from build123d import *

# Parameters (mm, degrees)
EXTRUDE1_DEPTH             = 500
SKETCH2_R                  = 1.75
EXTRUDE2_DEPTH             = 6.5
SKETCH_R                   = 3
SKETCH_R_2                 = 1.75
EXTRUDE4_DEPTH             = 3.5
CHAMFER1_SIZE              = 0.2
LPATTERN1_COUNT            = 24
LPATTERN1_PITCH            = 20
CHAMFER1_OF_LPATTERN1_SIZE = 0.2


with BuildPart() as part:
    # Sketch1 → Extrude1 (new body)
    with BuildSketch(Plane.XY):
        with BuildLine():
            Line((-4.3, -3.25), (4.3, -3.25))
            Line((4.3, -3.25), (4.5, -3.05))
            Line((4.5, -3.05), (4.5, 0.455012563))
            ThreePointArc((4.5, 0.455012563), (3.924845827, 0.712323349), (3.617735397, 1.2625))
            Line((3.617735397, 1.2625), (3.15008224, 1.2625))
            Line((3.15008224, 1.2625), (3.15008224, 1.7625))
            Line((3.15008224, 1.7625), (3.65008224, 1.7625))
            ThreePointArc((3.65008224, 1.7625), (3.973877727, 2.229724887), (4.5, 2.444987437))
            Line((4.5, 2.444987437), (4.5, 3.05))
            Line((4.5, 3.05), (4.3, 3.25))
            Line((4.3, 3.25), (-4.3, 3.25))
            Line((-4.3, 3.25), (-4.5, 3.05))
            Line((-4.5, 3.05), (-4.5, 2.444987437))
            ThreePointArc((-4.5, 2.444987437), (-3.973877727, 2.229724887), (-3.65008224, 1.7625))
            Line((-3.65008224, 1.7625), (-3.15008224, 1.7625))
            Line((-3.15008224, 1.7625), (-3.15008224, 1.2625))
            Line((-3.15008224, 1.2625), (-3.617735397, 1.2625))
            ThreePointArc((-3.617735397, 1.2625), (-3.924845827, 0.712323349), (-4.5, 0.455012563))
            Line((-4.5, 0.455012563), (-4.5, -3.05))
            Line((-4.5, -3.05), (-4.3, -3.25))
        make_face()
    extrude(amount=EXTRUDE1_DEPTH)

    # Sketch2 → Extrude2 (cut)
    with BuildSketch(Plane(origin=(0, 3.25, 0), x_dir=(1, 0, 0), z_dir=(0, 1, 0))):
        with Locations((0, -15)):
            Circle(SKETCH2_R)
    extrude2 = extrude(amount=-EXTRUDE2_DEPTH, mode=Mode.SUBTRACT)

    # Sketch → Extrude4 (cut)
    with BuildSketch(Plane(origin=(0, 3.25, 0), x_dir=(1, 0, 0), z_dir=(0, 1, 0))):
        with Locations((0, -15)):
            Circle(SKETCH_R)
        with Locations((0, -15)):
            Circle(SKETCH_R_2, mode=Mode.SUBTRACT)
    extrude4 = extrude(amount=-EXTRUDE4_DEPTH, mode=Mode.SUBTRACT)

    # Chamfer1
    chamfer1_edges = [part.edges().sort_by_distance(p)[0] for p in [
        (-1.75, -3.25, 15),
        (-3, 3.25, 15),
    ]]
    chamfer(chamfer1_edges, length=CHAMFER1_SIZE)

    # LPattern1: Extrude2, Extrude4 ×24
    with Locations(*[(0, 0, i * LPATTERN1_PITCH) for i in range(1, LPATTERN1_COUNT)]):
        add(extrude2, mode=Mode.SUBTRACT)
        add(extrude4, mode=Mode.SUBTRACT)

    # Chamfer1 of LPattern1
    chamfer1_of_lpattern1_edges = [part.edges().sort_by_distance(p)[0] for p in [
        (-1.75, -3.25, 35),
        (-3, 3.25, 35),
        (-1.75, -3.25, 55),
        (-3, 3.25, 55),
        (-1.75, -3.25, 75),
        (-3, 3.25, 75),
        (-1.75, -3.25, 95),
        (-3, 3.25, 95),
        (-1.75, -3.25, 115),
        (-3, 3.25, 115),
        (-1.75, -3.25, 135),
        (-3, 3.25, 135),
        (-1.75, -3.25, 155),
        (-3, 3.25, 155),
        (-1.75, -3.25, 175),
        (-3, 3.25, 175),
        (-1.75, -3.25, 195),
        (-3, 3.25, 195),
        (-1.75, -3.25, 215),
        (-3, 3.25, 215),
        (-1.75, -3.25, 235),
        (-3, 3.25, 235),
        (-1.75, -3.25, 255),
        (-3, 3.25, 255),
        (-1.75, -3.25, 275),
        (-3, 3.25, 275),
        (-1.75, -3.25, 295),
        (-3, 3.25, 295),
        (-1.75, -3.25, 315),
        (-3, 3.25, 315),
        (-1.75, -3.25, 335),
        (-3, 3.25, 335),
        (-1.75, -3.25, 355),
        (-3, 3.25, 355),
        (-1.75, -3.25, 375),
        (-3, 3.25, 375),
        (-1.75, -3.25, 395),
        (-3, 3.25, 395),
        (-1.75, -3.25, 415),
        (-3, 3.25, 415),
        (-1.75, -3.25, 435),
        (-3, 3.25, 435),
        (-1.75, -3.25, 455),
        (-3, 3.25, 455),
        (-1.75, -3.25, 475),
        (-3, 3.25, 475),
    ]]
    chamfer(chamfer1_of_lpattern1_edges, length=CHAMFER1_OF_LPATTERN1_SIZE)


solid = part.part
The model under review builds one solid part; all positions refer to its coordinate system, in mm. Round coordinates to 2 decimals unless told otherwise and drop trailing zeros. Write item = value, one per line. Start each with the question number.
Item 1: Insertion check: pin 1 (4.5 mm diameter, centred on x = 0, z = 235, fed in from +Y). The pin has a flat end and moves straight along its axis. Give the tip position at first contact, or say it passes through.
Item 2: Take a section at A-A on y = -1.5. Count the separate pieces of the cut face and the enclosed holes in it, plus the area to 3 significant figures.
Item 3: To check wall thickness, follow L1, parallel to X at y = -0.5, z = 335; L2, parallel to X at y = 1.95, z = 475; L3, parallel to Y at x = 4.25, z = 258.5. State the ranges of each line that lie inside material, in increasing order.
Result:
q1.pin_1 = -0.25
q2.separate_pieces = 1
q2.enclosed_holes = 24
q2.area = 4,270 mm²
q3.L1 = -4.5 to -1.75, 1.75 to 4.5
q3.L2 = -3.73 to -3, 3 to 3.73
q3.L3 = -3.25 to 0.51, 2.39 to 3.25
